```python
from build123d import *

# Parameters (mm, degrees)
SKETCH1_W                = 136
SKETCH1_H                = 122
BOSS_EXTRUDE1_DEPTH      = 80
FILLET1_R                = 20
SHELL1_T                 = -4
SHELL1_THICKNESS_2_DEPTH = 1
CUT_EXTRUDE2_DEPTH       = 5
F_4_CLEARANCE_HOLE1_D    = 3.2639
CUT_EXTRUDE3_DEPTH       = 66.75


with BuildPart() as part:
    # Sketch1 → Boss-Extrude1 (new body)
    with BuildSketch(Plane(origin=(0, 0, 0), x_dir=(1, 0, 0), z_dir=(0, 1, 0))):
        Rectangle(SKETCH1_W, SKETCH1_H)
    extrude(amount=BOSS_EXTRUDE1_DEPTH)

    # Fillet1
    fillet1_edges = [part.edges().sort_by_distance(p)[0] for p in [
        (68, 40, 61),
        (-68, 40, 61),
        (-68, 40, -61),
        (68, 40, -61),
    ]]
    fillet(fillet1_edges, radius=FILLET1_R)

    # Shell1
    shell1_openings = [part.faces().sort_by_distance(p)[0] for p in [
        (0, 80, 0),
    ]]
    offset(amount=SHELL1_T, openings=shell1_openings, kind=Kind.INTERSECTION)

    # Shell1 thickness 2 face (on inner face of the shell) → Shell1 thickness 2 (cut)
    with BuildSketch(Plane(origin=(0, 4, 0), x_dir=(0, 0, -1), z_dir=(0, -1, 0))):
        with BuildLine():
            ThreePointArc((57, -48), (52.313708499, -59.313708499), (41, -64))
            Line((41, -64), (-41, -64))
            ThreePointArc((-41, -64), (-52.313708499, -59.313708499), (-57, -48))
            Line((-57, -48), (-57, 48))
            ThreePointArc((-57, 48), (-52.313708499, 59.313708499), (-41, 64))
            Line((-41, 64), (41, 64))
            ThreePointArc((41, 64), (52.313708499, 59.313708499), (57, 48))
            Line((57, 48), (57, -48))
        make_face()
    extrude(amount=SHELL1_THICKNESS_2_DEPTH, mode=Mode.SUBTRACT)

    # Sketch5 → Cut-Extrude2 (cut)
    with BuildSketch(Plane(origin=(0, 80, 0), x_dir=(1, 0, 0), z_dir=(0, 1, 0))):
        with BuildLine():
            Line((48, 59.4), (-48, 59.4))
            ThreePointArc((-48, 59.4), (-61.010764774, 54.010764774), (-66.4, 41))
            Line((-66.4, 41), (-66.4, -41))
            ThreePointArc((-66.4, -41), (-61.010764774, -54.010764774), (-48, -59.4))
            Line((-48, -59.4), (48, -59.4))
            ThreePointArc((48, -59.4), (61.010764774, -54.010764774), (66.4, -41))
            Line((66.4, -41), (66.4, 41))
            ThreePointArc((66.4, 41), (61.010764774, 54.010764774), (48, 59.4))
        make_face()
        with BuildLine():
            Line((48, 57), (-48, 57))
            ThreePointArc((-48, 57), (-59.313708499, 52.313708499), (-64, 41))
            Line((-64, 41), (-64, -41))
            ThreePointArc((-64, -41), (-59.313708499, -52.313708499), (-48, -57))
            Line((-48, -57), (48, -57))
            ThreePointArc((48, -57), (59.313708499, -52.313708499), (64, -41))
            Line((64, -41), (64, 41))
            ThreePointArc((64, 41), (59.313708499, 52.313708499), (48, 57))
        make_face(mode=Mode.SUBTRACT)
    extrude(amount=-CUT_EXTRUDE2_DEPTH, mode=Mode.SUBTRACT)

    # #4 Clearance Hole1 (through all)
    with Locations(Plane(origin=(0, 3, 0), x_dir=(1, 0, 0), z_dir=(0, 1, 0))):
        with Locations((-25.4, 0), (25.4, 0)):
            Hole(F_4_CLEARANCE_HOLE1_D / 2)

    # Sketch8 → Cut-Extrude3 (cut)
    with BuildSketch(Plane(origin=(0, 80, 0), x_dir=(1, 0, 0), z_dir=(0, 1, 0))):
        Polygon((42, 61), (-42, 61), (-42, 59.4), (-46, 59.4), (-46, 57), (46, 57), (46, 59.4), (42, 59.4), align=None)
    extrude(amount=-CUT_EXTRUDE3_DEPTH, mode=Mode.SUBTRACT)


solid = part.part
```
The listing builds one solid part. Answer for the finished solid, in the listing's coordinates (mm). A direction names the side the tool comes from. Round coordinates to 2 decimals unless told otherwise and drop trailing zeros. Loops run counter-clockwise (first coordinate to the right, second up) from the corner with the lowest first, then second, coordinate; pieces in that order, holes last. Notation, with made-up numbers: (-3.5, -38) - (19.5, -38) arc R16 cw to (19.5, -14) - close; hole circle Ø1 at (-18, 33.5). An arc over 180 degrees is marked (long way). Use one line per item in the form item = value. Start each with the question number.
1. A tool of negligible diameter and unlimited length cuts with its end or side. For faces 1 (the face through (66.4, 78, 1)), 2 (the face through (26.695, 1.479, 0.993)), from which of +Z, -Z, +X, -X, +Y, -Y can it reach the whole face along a straight path? Write none if from no direction.
2. Given pin 1 Ø1.5 at (x, z) = (51, 13) entering from -Y; pin 2 Ø1 at (x, z) = (36.5, 11) entering from +Y; pin 3 Ø2.5 at (x, y) = (-21.5, 78.5) entering from -Z; pin 4 Ø4.5 at (x, z) = (-18, -59.5) entering from +Y, each flat-ended and moving along its own axis, determine where each tip first touches the part or whether it passes through.
3. The part is cut by section A-A on x = 25.4. Determine the outline of the cut face in (y, z).
4. The part is cut by section D-D on y = 47.5. Determine the outline of the cut face in (x, z).
5. For a pull along Z with two mould halves and no side action, classify faces 3 (the face through (-1, 0, -1)), 4 (the face through (-62.297, 40.56, -54.986)), 5 (the face through (-64, 38, 1)) as pulls with the +Z half, pulls with the -Z half, needs draft (parallel to the pull), parting line crosses it, or undercut.
6. Consider line 1 (Z direction, x = -10, y = 5); line 2 (Z direction, x = 25.4, y = 1.75); line 3 (X direction, y = 43, z = -37). Determine where each line is inside the solid, lowest interval first. Write a range as [from, to].
7. The part is cut by section B-B on z = 0. Determine the outline of the cut face in (x, y), then the cut area to 3 significant figures.
8. The part is cut by section C-C on y = 10. Determine the outline of the cut face in (x, z).
Geometry check:
q1.face_1 = +Y
q1.face_2 = +Y, -Y
q2.pin_1 = 0
q2.pin_2 = 3
q2.pin_3 = 59.4
q2.pin_4 = 13.25
q3.outline = (0, -61) - (13.25, -61) - (13.25, -57) - (3, -57) - (3, -1.63) - (0, -1.63) - close; (0, 1.63) - (3, 1.63) - (3, 57) - (75, 57) - (75, 59.4) - (80, 59.4) - (80, 61) - (0, 61) - close
q4.outline = (-68, -41) arc R20 ccw to (-48, -61) - (-42, -61) - (-42, -59.4) - (-46, -59.4) - (-46, -57) - (-48, -57) arc R16 cw to (-64, -41) - (-64, 41) arc R16 cw to (-48, 57) - (48, 57) arc R16 cw to (64, 41) - (64, -41) arc R16 cw to (48, -57) - (46, -57) - (46, -59.4) - (42, -59.4) - (42, -61) - (48, -61) arc R20 ccw to (68, -41) - (68, 41) arc R20 ccw to (48, 61) - (-48, 61) arc R20 ccw to (-68, 41) - close
q5.face_3 = needs draft
q5.face_4 = pulls with the -Z half
q5.face_5 = undercut
q6.line_1 = [-61, -57], [57, 61]
q6.line_2 = [-61, -1.63], [1.63, 61]
q6.line_3 = [-68, -64], [64, 68]
q7.outline = (-68, 0) - (-27.03, 0) - (-27.03, 3) - (-64, 3) - (-64, 75) - (-66.4, 75) - (-66.4, 80) - (-68, 80) - close; (-23.77, 0) - (23.77, 0) - (23.77, 3) - (-23.77, 3) - close; (27.03, 0) - (68, 0) - (68, 80) - (66.4, 80) - (66.4, 75) - (64, 75) - (64, 3) - (27.03, 3) - close
q7.area = 980 mm^2
q8.outline = (-68, -41) arc R20 ccw to (-48, -61) - (48, -61) arc R20 ccw to (68, -41) - (68, 41) arc R20 ccw to (48, 61) - (-48, 61) arc R20 ccw to (-68, 41) - close; hole (-64, -41) arc R16 ccw to (-48, -57) - (48, -57) arc R16 ccw to (64, -41) - (64, 41) arc R16 ccw to (48, 57) - (-48, 57) arc R16 ccw to (-64, 41) - close
